The listing builds one solid part. Answer for the finished solid, in the listing's coordinates (mm). A direction names the side the tool comes from. Round coordinates to 2 decimals unless told otherwise and drop trailing zeros. Loops run counter-clockwise (first coordinate to the right, second up) from the corner with the lowest first, then second, coordinate; pieces in that order, holes last. Notation, with made-up numbers: M 83.5,-2 L 112.5,-2 A23 ccw 112.5,21 Z; hole C -30,-33.5 d10. An arc over 180 degrees is marked long. Answer as a JSON object with one key per item and string values.
Autodesk Inventor part; units mm, degrees
ref_plane "YZ Plane" through (0, 0, 0) normal (1, 0, 0) x (0, 1, 0)
ref_plane "XZ Plane" through (0, 0, 0) normal (0, 1, 0) x (-1, 0, 0)
ref_plane "XY Plane" through (0, 0, 0) normal (0, 0, 1) x (1, 0, 0)
sketch "Sketch1" plane through (0, 0, 0) normal (0, 1, 0) x (-1, 0, 0)
  line L0 (0, 25.4) -> (25.4, 25.4)
  line L1 (25.4, 25.4) -> (25.4, 0)
  line L2 (25.4, 0) -> (0, 0)
  line L3 (0, 0) -> (0, 25.4)
  line L4 (22.225, 22.225) -> (3.175, 22.225)
  line L5 (3.175, 22.225) -> (3.175, 3.175)
  line L6 (3.175, 3.175) -> (22.225, 3.175)
  line L7 (22.225, 3.175) -> (22.225, 22.225)
  dimension "d0" = 25.4
  dimension "d1" = 25.4
  dimension "d2" = 3.175
extrude "Extrusion1" add sketch "Sketch1" along normal blind 660.4
sketch "Sketch2" plane through (-25.4, 0, 25.4) normal (0, 0, 1) x (1, 0, 0)
  line L0 (25.4, 0) -> (0, 0)
  line L1 (0, 660.4) -> (25.4, 660.4)
  line L2 (12.7, 660.4) -> (12.7, 0) construction
  circle A0 centre (12.7, 38.1) radius 2.8575
  circle A1 centre (12.7, 63.5) radius 2.8575
  circle A2 centre (12.7, 88.9) radius 2.8575
  circle A3 centre (12.7, 114.3) radius 2.8575
  circle A4 centre (12.7, 139.7) radius 2.8575
  circle A5 centre (12.7, 165.1) radius 2.8575
  circle A6 centre (12.7, 190.5) radius 2.8575
  circle A7 centre (12.7, 215.9) radius 2.8575
  circle A8 centre (12.7, 241.3) radius 2.8575
  circle A9 centre (12.7, 266.7) radius 2.8575
  circle A10 centre (12.7, 292.1) radius 2.8575
  circle A11 centre (12.7, 317.5) radius 2.8575
  circle A12 centre (12.7, 342.9) radius 2.8575
  circle A13 centre (12.7, 368.3) radius 2.8575
  circle A14 centre (12.7, 393.7) radius 2.8575
  circle A15 centre (12.7, 419.1) radius 2.8575
  circle A16 centre (12.7, 444.5) radius 2.8575
  circle A17 centre (12.7, 469.9) radius 2.8575
  circle A18 centre (12.7, 495.3) radius 2.8575
  circle A19 centre (12.7, 520.7) radius 2.8575
  circle A20 centre (12.7, 546.1) radius 2.8575
  circle A21 centre (12.7, 571.5) radius 2.8575
  circle A22 centre (12.7, 596.9) radius 2.8575
  circle A23 centre (12.7, 622.3) radius 2.8575
  dimension "d5" = 5.715
  dimension "d6" = 38.1
  dimension "d7" = 660.4
  dimension "d10" = 25.4
extrude "Extrusion2" cut sketch "Sketch2" against normal through all contours A0 | A1 | A5 | A6 | A11 | A12 | A17 | A18 | A22 | A23
sketch "Sketch3" plane through (-25.4, 0, 0) normal (-1, 0, 0) x (0, 0, 1)
  line L0 (25.4, 0) -> (0, 0)
  line L1 (0, 660.4) -> (25.4, 660.4)
  line L2 (12.7, 660.4) -> (12.7, 0) construction
  circle A0 centre (12.7, 552.45) radius 3.302
  circle A1 centre (12.7, 107.95) radius 3.302
  circle A2 centre (12.7, 650.875) radius 3.302
  circle A3 centre (12.7, 635) radius 3.302
  circle A4 centre (12.7, 25.4) radius 3.302
  circle A5 centre (12.7, 9.525) radius 3.302
  circle A6 centre (12.7, 520.7) radius 3.302
  circle A7 centre (12.7, 495.3) radius 3.302
  circle A8 centre (12.7, 469.9) radius 3.302
  circle A9 centre (12.7, 444.5) radius 3.302
  circle A10 centre (12.7, 419.1) radius 3.302
  circle A11 centre (12.7, 393.7) radius 3.302
  circle A12 centre (12.7, 368.3) radius 3.302
  circle A13 centre (12.7, 342.9) radius 3.302
  circle A14 centre (12.7, 317.5) radius 3.302
  circle A15 centre (12.7, 292.1) radius 3.302
  circle A16 centre (12.7, 266.7) radius 3.302
  circle A17 centre (12.7, 241.3) radius 3.302
  circle A18 centre (12.7, 215.9) radius 3.302
  circle A19 centre (12.7, 190.5) radius 3.302
  circle A20 centre (12.7, 165.1) radius 3.302
  circle A21 centre (12.7, 139.7) radius 3.302
  dimension "d34" = 16
  dimension "d27" = 6.604
  dimension "d28" = 6.604
  dimension "d29" = 107.95
  dimension "d30" = 107.95
  dimension "d31" = 444.5
  dimension "d32" = 31.75
  dimension "d33" = 6.604
  dimension "d36" = 25.4
extrude "Extrusion3" cut sketch "Sketch3" against normal blind 25.4
sketch "Sketch4" plane through (0, 0, 25.4) normal (1, 0, 0) x (0, 0, -1)
  circle A0 centre (12.7, 25.4) radius 3.302
  circle A1 centre (12.7, 635) radius 3.302
  line L0 (25.4, 0) -> (0, 0)
  line L1 (0, 660.4) -> (25.4, 660.4)
  line L2 (12.7, 660.4) -> (12.7, 0) construction
  circle A2 centre (12.7, 50.8) radius 3.302
  circle A3 centre (12.7, 69.85) radius 3.302
  circle A4 centre (12.7, 609.6) radius 3.302
  circle A5 centre (12.7, 590.55) radius 3.302
  dimension "d41" = 25.4
  dimension "d42" = 19.05
  dimension "d43" = 6.604
  dimension "d45" = 25.4
  dimension "d46" = 19.05
extrude "Extrusion4" cut sketch "Sketch4" against normal blind 25.4 contours A2 | A3 | A4 | A5
equation "\"d27\" = d28"
equation "\"d30\" = d29"
equation "\"d33\" = d28"
properties part number "Chassis V1.500 Part2" material "Aluminum 6061"
Item 1: Straight lines are drawn through the part: line 1 (Z direction, x = -1.9, y = 190.5); line 2 (Z direction, x = -21, y = 29) (3 decimals); line 3 (X direction, y = 194, z = 7.5) (3 decimals). For each, find the intervals that lie inside material, in ascending order.
Values follow:
{"line 1": "0 to 9.4, 16 to 25.4", "line 2": "0 to 3.175, 22.225 to 25.4", "line 3": "-25.4 to -22.225, -3.175 to 0"}
Item 2: Determine the mould class of faces 1 (the face through (-24, 0, 13)), 2 (the face through (-13, 326, 0)), 3 (the face through (-13, 326, 3.175)), 4 (the face through (-13, 326, 25.4)) for opening direction Z: released by +Z, released by -Z, zero draft, split by the parting line, or undercut.
Values follow:
{"face 1": "zero draft", "face 2": "released by -Z", "face 3": "undercut", "face 4": "released by +Z"}
Item 3: A flat-ended cylindrical pin translates along its axis: P1, Ø6, axis at y = 25.4, z = 12.7, coming from the +X side. Find the tip coordinate at first contact, or state that the pin passes through.
Values follow:
{"P1": "through"}
Item 4: Which of the six approach directions +Z, -Z, +X, -X, +Y, -Y give full straight-line access (tool end or side, diameter ignored) to faces 5 (the face through (-3.175, 326, 13)), 6 (the face through (-25.4, 326, 13))?
Values follow:
{"face 5": "+Y, -Y", "face 6": "+Z, -Z, -X, +Y, -Y"}
Item 5: The part is cut by section A-A (y = 97). Give the vertices of the cut face in (x, z) (3 decimals), then the cut area to 3 significant figures.
Values follow:
{"outline": "M -25.4,0 L 0,0 L 0,25.4 L -25.4,25.4 Z; hole M -22.225,3.175 L -3.175,3.175 L -3.175,22.225 L -22.225,22.225 Z", "area": "282 mm^2"}
